CAD build for the part. Positions are in the model's coordinates, mm. A direction names the side the tool comes from. Coordinates: 2 decimals unless noted, no trailing zeros. Loops run counter-clockwise (first coordinate to the right, second up) from the corner with the lowest first, then second, coordinate; pieces in that order, holes last. Notation, with made-up numbers: (77, -18) -> (102, -18) arc R13 cw to (102, -6) -> close; hole circle Ø7 at (63, -39). An arc over 180 degrees is marked (long way). Write each question's results on one line, items separated by ' | '.
from build123d import *

# Parameters (mm, degrees)
CUT_EXTRUDE1_DEPTH = 5
CIRPATTERN1_COUNT  = 18
SKETCH4_R          = 1.5
CUT_EXTRUDE3_DEPTH = 5


with BuildPart() as part:
    # Sketch1 → Revolve2 (revolve)
    with BuildSketch(Plane.XY):
        Polygon((0, 4), (0, 80), (-10, 80), (-10, 15), (-25, 15), (-25, 4), align=None)
    revolve(axis=Axis((0, 0, 0), (-1, 0, 0)))

    # Sketch2 → Cut-Extrude1 (cut)
    with BuildSketch(Plane(origin=(0, 0, 0), x_dir=(0, 0, -1), z_dir=(1, 0, 0))):
        with BuildLine():
            Line((5, 50), (5, 80))
            Line((5, 80), (-5, 80))
            Line((-5, 80), (-5, 50))
            ThreePointArc((-5, 50), (0, 45), (5, 50))
        make_face()
    cut_extrude1 = extrude(amount=-CUT_EXTRUDE1_DEPTH, mode=Mode.SUBTRACT)

    # CirPattern1: Cut-Extrude1 ×18 about axis
    cirpattern1_axis = Axis((0, 0, 0), (1, 0, 0))
    for i in range(1, CIRPATTERN1_COUNT):
        add(cut_extrude1.rotate(cirpattern1_axis, i * 360 / CIRPATTERN1_COUNT), mode=Mode.SUBTRACT)

    # Sketch4 → Cut-Extrude3 (cut)
    with BuildSketch(Plane(origin=(0, 0, 0), x_dir=(0, 0, -1), z_dir=(1, 0, 0))):
        with Locations((-55.155199905, 46.280707897)):
            Circle(SKETCH4_R)
        with Locations((55.155199905, 46.280707897)):
            Circle(SKETCH4_R)
        with Locations((55.155199905, -46.280707897)):
            Circle(SKETCH4_R)
        with Locations((-55.155199905, -46.280707897)):
            Circle(SKETCH4_R)
        with Locations((0, 30)):
            Circle(SKETCH4_R)
        with Locations((30, 0)):
            Circle(SKETCH4_R)
        with Locations((0, -30)):
            Circle(SKETCH4_R)
        with Locations((-30, 0)):
            Circle(SKETCH4_R)
    extrude(amount=-CUT_EXTRUDE3_DEPTH, mode=Mode.SUBTRACT)


solid = part.part
1) Drill centre lines: L1, parallel to Y at x = -2.95, z = 0; L2, parallel to Z at x = -17.75, y = 0; L3, parallel to X at y = -14, z = -31. Where is each one in solid material? Low to high. Write a range as from..to.
Outcome:
L1: y = -45..-31.5, -28.5..-4, 4..28.5, 31.5..45 | L2: z = -15..-4, 4..15 | L3: x = -10..0
2) Pin check, flat tips, straight feed: pin 1 (12 mm diameter, centred on x = -15.5, z = 18.5, fed in from +Y); pin 2 (0.9 mm diameter, centred on y = -0.5, z = 30, fed in from +X); pin 3 (1.8 mm diameter, centred on y = -46.28, z = -55.16, fed in from -X). Stop position of each tip, or through.
Outcome:
pin 1: stops at y = 78.36 | pin 2: stops at x = -5 | pin 3: stops at x = -10
3) Which spindle directions (+Z, -Z, +X, -X, +Y, -Y) get a long thin tool onto all of the face, cutting with end or side? Do faces 3 (the cylindrical face through (-2.465, 22.596, -38.917)), 4 (the flat face through (-2, 65, -5)), 5 (the cylindrical face through (-2, -45, 0)). Say none if no direction does.
Outcome:
face 3: +X | face 4: +X, +Y | face 5: +X, -Y
4) Two-plate mould, pull along Z, no slides. Class faces 1 (the cylindrical face through (-2.465, -34.544, 28.842)), 2 (the cylindrical face through (-2.465, -7.706, -44.337)): pulls with the +Z half, pulls with the -Z half, needs draft (parallel to the pull), parting line crosses it, or undercut.
Outcome:
face 1: undercut | face 2: undercut
5) Slice it at C-C (x = -2.5). Count the separate pieces of the cut face and the enclosed holes in it, then the cut area to 3 significant figures.
Outcome:
separate pieces: 1 | enclosed holes: 9 | area: 13,900 mm^2
6) Slice it at B-B (x = -13.5). Write the cut outline in (y, z), then the cut area to 3 significant figures.
Outcome:
outline: circle Ø30 at (0, 0); hole circle Ø8 at (0, 0) | area: 657 mm^2
7) Slice it at A-A (y = -25). Write the cut outline in (x, z), then the cut area to 3 significant figures.
Outcome:
outline: (-10, -75.99) -> (0, -75.99) -> (0, -53.3) -> (-5, -53.3) -> (-5, -38.3) -> (0, -38.3) -> (0, 38.3) -> (-5, 38.3) -> (-5, 53.3) -> (0, 53.3) -> (0, 75.99) -> (-10, 75.99) -> close | area: 1,370 mm^2
